Here's the drawing with two shaded views (mm, measured from the low corner). I have some questions. Coordinates: 2 decimals unless noted, no trailing zeros. Write each loop counter-clockwise with the first axis right and the second up, starting at its lowest first coordinate (ties: lowest second). Pieces come first, ordered by that corner, then holes. Notation, with made-up numbers: (54, 30) - (82, 30) arc R24 ccw to (82, 63) - close; hole circle Ø8 at (45, -10). An arc over 180 degrees is marked (long way). Answer in a Markdown table with one row per item. Add a question column.
Item 1: I'm going to push flat-ended pins straight in: pin 1 (1 mm diameter, centred on x = 8.5, z = 4, fed in from -Y); pin 2 (2 mm diameter, centred on y = 3, z = 8, fed in from +X); pin 3 (3 mm diameter, centred on x = 6.5, z = 24, fed in from -Y). Where does each tip first touch, or does it pass through?
Item 2: Imagine slicing it at A-A (y = 4.8). Please give me the cut outline in (x, z).
Item 3: Imagine slicing it at C-C (z = 5). Please give me the cut outline in (x, y).
Item 4: If I drill on probe 1 along Y at (x, z) = (4.8, 16.75); probe 2 along Y at (x, z) = (3.25, 25.5); probe 3 along X at (y, z) = (7, 2.75), over which ranges is the centre line in solid material (lowest first)? Write a range as from..to.
Item 5: We'd pull the mould along Y, two halves only. Please class the marked faces 1, 2 and 3: +Y half, -Y half, draft (parallel to the pull), parting line (faces both ways), or undercut.
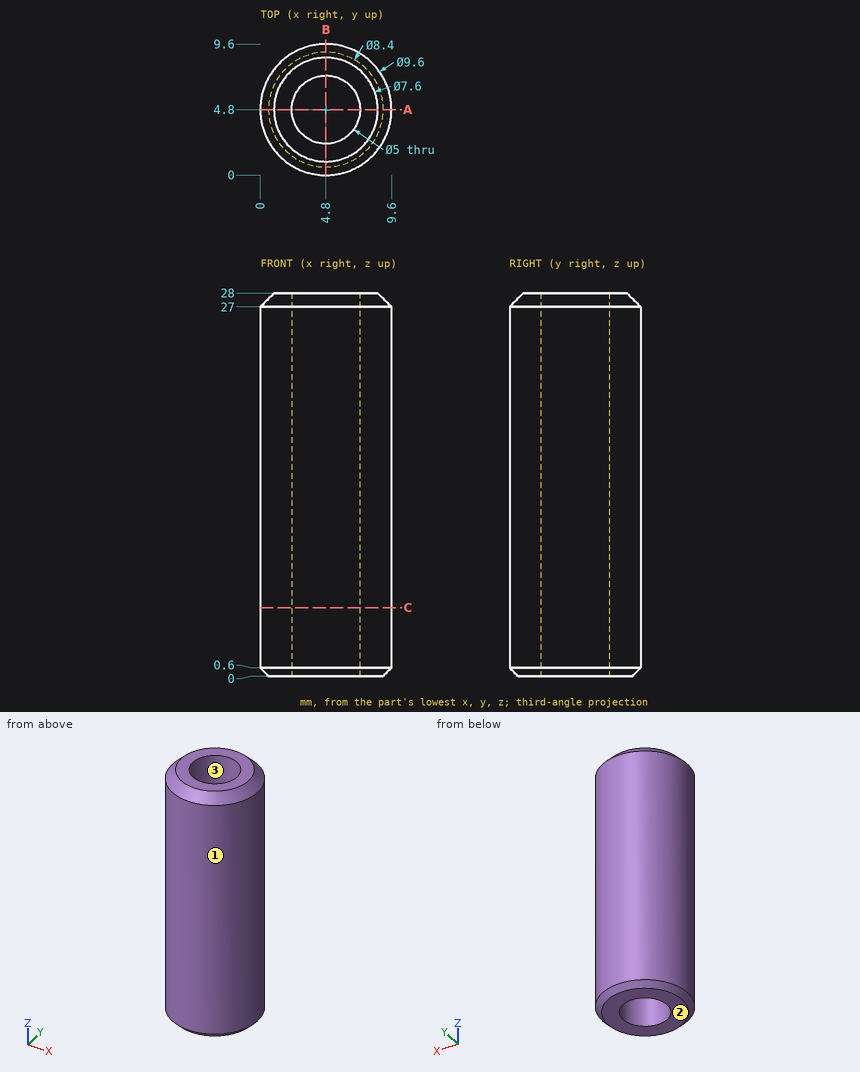
Here are the results:
| question | item | result |
|---|---|---|
| 1 | pin 1 | stops at y = 1.22 |
| 1 | pin 2 | stops at x = 9.53 |
| 1 | pin 3 | stops at y = 0 |
| 2 | outline | (0, 0.6) - (0.6, 0) - (2.3, 0) - (2.3, 28) - (1, 28) - (0, 27) - close; (7.3, 0) - (9, 0) - (9.6, 0.6) - (9.6, 27) - (8.6, 28) - (7.3, 28) - close |
| 3 | outline | circle Ø9.6 at (4.8, 4.8); hole circle Ø5 at (4.8, 4.8) |
| 4 | probe 1 | y = 0..2.3, 7.3..9.6 |
| 4 | probe 2 | y = 0.26..2.84, 6.76..9.34 |
| 4 | probe 3 | x = 0.53..3.61, 5.99..9.07 |
| 5 | face 1 | parting line |
| 5 | face 2 | draft |
| 5 | face 3 | undercut |
